from build123d import *

# Parameters (mm, degrees)
BOSS_EXTRUDE1_DEPTH = 200
CUT_EXTRUDE1_DEPTH  = 195
SKETCH5_R           = 1.65
SKETCH5_W           = 7.65
SKETCH5_H           = 20.2
CUT_EXTRUDE4_DEPTH  = 70
SKETCH7_R           = 4.5
SKETCH7_R_2         = 3
CUT_EXTRUDE6_DEPTH  = 70
FILLET1_R           = 4
CUT_EXTRUDE7_DEPTH  = 70
SKETCH10_R          = 1.6
CUT_EXTRUDE8_DEPTH  = 6
BOSS_EXTRUDE2_DEPTH = 20
SKETCH12_R          = 2
CUT_EXTRUDE9_DEPTH  = 10
SKETCH13_R          = 1.75
CUT_EXTRUDE10_DEPTH = 10


with BuildPart() as part:
    # Sketch1 → Boss-Extrude1 (new body)
    with BuildSketch(Plane(origin=(0, 0, 0), x_dir=(0, 0, -1), z_dir=(1, 0, 0))):
        Polygon((90, 0), (45, 77.942286341), (-45, 77.942286341), (-90, 0), (-45, -77.942286341), (45, -77.942286341), align=None)
    extrude(amount=BOSS_EXTRUDE1_DEPTH)

    # Sketch2 → Cut-Extrude1 (cut)
    with BuildSketch(Plane(origin=(200, 0, 0), x_dir=(0, 0, -1), z_dir=(1, 0, 0))):
        Polygon((84.226497308, 0), (42.113248654, 72.942286341), (-42.113248654, 72.942286341), (-84.226497308, 0), (-42.113248654, -72.942286341), (42.113248654, -72.942286341), align=None)
    extrude(amount=-CUT_EXTRUDE1_DEPTH, mode=Mode.SUBTRACT)

    # Sketch5 → Cut-Extrude4 (cut)
    with BuildSketch(Plane(origin=(0, -38.97114317, 67.5), x_dir=(1, 0, 0), z_dir=(0, -0.500000000000007, 0.8660254037844347))):
        with Locations(Location((68.825, 9.75, 0), (0, 0, 270))):
            Circle(SKETCH5_R)
        with Locations(Location((68.825, -19.75, 0), (0, 0, 270))):
            Circle(SKETCH5_R)
        with Locations((68.825, -5)):
            Rectangle(SKETCH5_W, SKETCH5_H)
    extrude(amount=-CUT_EXTRUDE4_DEPTH, mode=Mode.SUBTRACT)

    # Sketch7 → Cut-Extrude6 (cut)
    with BuildSketch(Plane(origin=(5, 0, 0), x_dir=(0, 0, -1), z_dir=(1, 0, 0))):
        Circle(SKETCH7_R)
        with Locations((60, 0)):
            Circle(SKETCH7_R_2)
        with Locations((30, 51.961524227)):
            Circle(SKETCH7_R_2)
        with Locations((-30, 51.961524227)):
            Circle(SKETCH7_R_2)
        with Locations((-60, 0)):
            Circle(SKETCH7_R_2)
        with Locations((-30, -51.961524227)):
            Circle(SKETCH7_R_2)
        with Locations((30, -51.961524227)):
            Circle(SKETCH7_R_2)
    extrude(amount=-CUT_EXTRUDE6_DEPTH, mode=Mode.SUBTRACT)

    # Fillet1
    fillet1_edges = [part.edges().sort_by_distance(p)[0] for p in [
        (5, -36.47114317, -63.169872981),
        (102.5, 0, -84.226497308),
        (5, -72.942286341, 0),
        (102.5, -72.942286341, -42.113248654),
        (5, -36.47114317, 63.169872981),
        (102.5, -72.942286341, 42.113248654),
        (5, 36.47114317, 63.169872981),
        (5, 72.942286341, 0),
        (102.5, 72.942286341, 42.113248654),
        (5, 36.47114317, -63.169872981),
        (102.5, 72.942286341, -42.113248654),
    ]]
    fillet(fillet1_edges, radius=FILLET1_R)

    # Sketch9 → Cut-Extrude7 (cut)
    with BuildSketch(Plane(origin=(200, 0, 0), x_dir=(0, 0, -1), z_dir=(1, 0, 0))):
        Polygon((45, 77.942286341), (90, 0), (45, -77.942286341), (-45, -77.942286341), (-90, 0), (-45, 77.942286341), align=None)
    extrude(amount=-CUT_EXTRUDE7_DEPTH, mode=Mode.SUBTRACT)

    # Sketch10 → Cut-Extrude8 (cut)
    with BuildSketch(Plane(origin=(0, 38.97114317, 67.5), x_dir=(1, 0, 0), z_dir=(0, 0.49999999999999495, 0.8660254037844417))):
        with Locations(Location((110, -5, 0), (0, 0, 270))):
            Circle(SKETCH10_R)
        with Locations(Location((121, -5, 0), (0, 0, 270))):
            Circle(SKETCH10_R)
    extrude(amount=-CUT_EXTRUDE8_DEPTH, mode=Mode.SUBTRACT)

    # Sketch11 → Boss-Extrude2 (add)
    with BuildSketch(Plane.ZY):
        Polygon((90, 0), (45, 77.942286341), (-45, 77.942286341), (-90, 0), (-45, -77.942286341), (45, -77.942286341), align=None)
        Polygon((84.226497308, 0), (42.113248654, 72.942286341), (-42.113248654, 72.942286341), (-84.226497308, 0), (-42.113248654, -72.942286341), (42.113248654, -72.942286341), align=None, mode=Mode.SUBTRACT)
    extrude(amount=BOSS_EXTRUDE2_DEPTH)

    # Sketch12 → Cut-Extrude9 (cut)
    with BuildSketch(Plane(origin=(0, 77.942286341, 0), x_dir=(1, 0, 0), z_dir=(0, 1, 0))):
        with Locations(Location((100.87, 0, 0), (0, 0, 270))):
            Circle(SKETCH12_R)
        with Locations(Location((37.37, 0, 0), (0, 0, 270))):
            Circle(SKETCH12_R)
    extrude(amount=-CUT_EXTRUDE9_DEPTH, mode=Mode.SUBTRACT)

    # Sketch13 → Cut-Extrude10 (cut)
    with BuildSketch(Plane(origin=(0, 38.97114317, 67.5), x_dir=(1, 0, 0), z_dir=(0, 0.49999999999999983, 0.8660254037844387))):
        with Locations(Location((70.766818174, 1.341454493, 0), (0, 0, 270))):
            Circle(SKETCH13_R)
        with Locations(Location((38.766818174, 1.341454493, 0), (0, 0, 270))):
            Circle(SKETCH13_R)
    extrude(amount=-CUT_EXTRUDE10_DEPTH, mode=Mode.SUBTRACT)


solid = part.part
Geometry: final body of the model. Coordinates: model frame, mm. A direction names the side the tool comes from. Coordinates: 2 decimals unless noted, no trailing zeros. Order: outer loops, then holes, each group sorted by start corner. A loop starts at its lowest first (then second) coordinate and runs counter-clockwise, first axis right, second up.
1) Ray query, probe 1 along Y at (x, z) = (2.75, 0); probe 2 along Y at (x, z) = (62.5, -39.5); probe 3 along X at (y, z) = (-30, -51.5). Return the intervals inside material, ascending.
Result sheet:
probe 1: y = -77.94 to -4.5, 4.5 to 77.94
probe 2: y = -77.94 to -72.94, 72.94 to 77.94
probe 3: x = 0 to 5
2) Section C-C (z = -15). Return loops of the section in (x, y), then the cut area to 3 significant figures.
Result sheet:
outline: (-20, -77.94) - (130, -77.94) - (130, -72.94) - (9, -72.94) arc R4 cw to (5, -68.94) - (5, 68.94) arc R4 cw to (9, 72.94) - (130, 72.94) - (130, 77.94) - (-20, 77.94) - (-20, 72.94) - (0, 72.94) - (0, -72.94) - (-20, -72.94) - close
area: 2,240 mm2
3) Draft query along Y for faces 4 (the flat face through (70, 72.942, -1)), 5 (the flat face through (56, 77.942, 1)). Return one class per face: released by +Y, released by -Y, zero draft, split by the parting line, or undercut.
Result sheet:
face 4: undercut
face 5: released by +Y
4) Set-up query: faces 1 (the flat face through (68.77, -50.82, 57.82)), 2 (the flat face through (-9.86, 35.961, 63.465)), 3 (the flat face through (70.347, -27.092, 68.585)). Return all of +Z, -Z, +X, -X, +Y, -Y with unobstructed straight access to the full face (end or side cutting, diameter ignored); none if empty.
Result sheet:
face 1: +Z
face 2: -X
face 3: +X
5) First-contact query: P1, Ø1, axis at y = 37.5, z = -14, coming from the +X side; P2, Ø6, axis at x = 45, z = -66.5, coming from the +Y side; P3, Ø4, axis at x = 83.5, z = 53.5, coming from the -Y side; P4, Ø5, axis at y = 0, z = -60, coming from the -X side. Flat tips, straight axial feed; report the tip coordinate or a pass-through.
Result sheet:
P1: stops at x = 5
P2: stops at y = 45.9
P3: stops at y = -66.68
P4: passes through
6) Section B-B (z = 30). Return loops of the section in (x, y).
Result sheet:
outline: (-20, -77.94) - (130, -77.94) - (130, -72.94) - (9, -72.94) arc R4 cw to (5, -68.94) - (5, -54.96) - (0, -54.96) - (0, -72.94) - (-20, -72.94) - close; (-20, 72.94) - (0, 72.94) - (0, 54.96) - (5, 54.96) - (5, 68.94) arc R4 cw to (9, 72.94) - (130, 72.94) - (130, 77.94) - (-20, 77.94) - close; (0, -48.96) - (5, -48.96) - (5, 48.96) - (0, 48.96) - close
7) Section A-A (x = 106). Return loops of the section in (y, z), then the cut area to 3 significant figures.
Result sheet:
outline: (-77.94, -45) - (0, -90) - (77.94, -45) - (77.94, 45) - (0, 90) - (-77.94, 45) - close; hole (-72.94, -39.8) arc R4 ccw to (-70.94, -43.27) - (-2, -83.07) arc R4 ccw to (2, -83.07) - (70.94, -43.27) arc R4 ccw to (72.94, -39.8) - (72.94, 39.8) arc R4 ccw to (70.94, 43.27) - (0, 84.23) - (-70.94, 43.27) arc R4 ccw to (-72.94, 39.8) - close
area: 2,620 mm2
